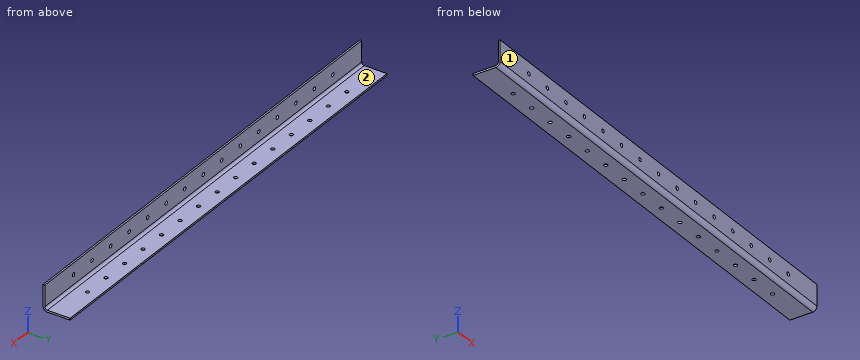
from build123d import *

# Parameters (mm, degrees)
SKETCH1_W                    = 2600
SKETCH1_H                    = 150
BASE_FLANGE1_DEPTH           = 10
EDGE_FLANGE1_STRIP_W         = 68
EDGE_FLANGE1_STRIP_H         = 10
EDGE_FLANGE1_STRIP_CUT_DEPTH = 2600
EDGE_FLANGE1_DEPTH           = 2600
SKETCH12_R                   = 10
CUT_EXTRUDE1_DEPTH           = 10
SKETCH13_R                   = 10
CUT_EXTRUDE2_DEPTH           = 10
LPATTERN1_COUNT              = 15
LPATTERN1_PITCH              = 152


# Sheet-metal steps are written as plain solids
with BuildPart() as part:
    # Sketch1 → Base-Flange1 (new body)
    with BuildSketch(Plane.XY):
        Rectangle(SKETCH1_W, SKETCH1_H)
    extrude(amount=-BASE_FLANGE1_DEPTH)

    # Edge-Flange1 strip (across the edge) → Edge-Flange1 strip cut (cut)
    with BuildSketch(Plane(origin=(-1300, -75, 0), x_dir=(0, 1, 0), z_dir=(1, 0, 0))):
        with Locations((-10, -5)):
            Rectangle(EDGE_FLANGE1_STRIP_W, EDGE_FLANGE1_STRIP_H)
    extrude(amount=EDGE_FLANGE1_STRIP_CUT_DEPTH, mode=Mode.SUBTRACT)

    # Edge-Flange1 section (across the edge) → Edge-Flange1 (add)
    with BuildSketch(Plane(origin=(-1300, -75, 0), x_dir=(0, 1, 0), z_dir=(1, 0, 0))):
        with BuildLine():
            Line((0, 14), (0, 130))
            Line((0, 130), (10, 130))
            Line((10, 130), (10, 14))
            ThreePointArc((10, 14), (14.100505063, 4.100505063), (24, 0))
            Line((24, 0), (24, -10))
            ThreePointArc((24, -10), (7.029437252, -2.970562748), (0, 14))
        make_face()
    extrude(amount=EDGE_FLANGE1_DEPTH)

    # Sketch12 → Cut-Extrude1 (cut)
    with BuildSketch(Plane(origin=(0, -75, 0), x_dir=(-1, 0, 0), z_dir=(0, -1, 0))):
        with Locations(Location((1064, -67, 0), (0, 0, 90))):
            Circle(SKETCH12_R)
    cut_extrude1 = extrude(amount=-CUT_EXTRUDE1_DEPTH, mode=Mode.SUBTRACT)

    # Sketch13 → Cut-Extrude2 (cut)
    with BuildSketch(Plane(origin=(0, 0, -10), x_dir=(-1, 0, 0), z_dir=(0, 0, -1))):
        with Locations((1064, 12)):
            Circle(SKETCH13_R)
    cut_extrude2 = extrude(amount=-CUT_EXTRUDE2_DEPTH, mode=Mode.SUBTRACT)

    # LPattern1: Cut-Extrude1, Cut-Extrude2 ×15
    with Locations(*[(i * LPATTERN1_PITCH, 0, 0) for i in range(1, LPATTERN1_COUNT)]):
        add(cut_extrude1, mode=Mode.SUBTRACT)
        add(cut_extrude2, mode=Mode.SUBTRACT)


solid = part.part
For this review, take the finished solid that the model builds, in its own axes (mm). Face numbers are marked on the shaded views. A direction names the side the tool comes from. Give positions to 0.01 mm unless a question says otherwise; leave off trailing zeros. Order: outer loops, then holes, each group sorted by start corner. A loop starts at its lowest first (then second) coordinate and runs counter-clockwise, first axis right, second up. Notation, with made-up numbers: M 21.5,43 L 28.5,43 A21 cw 28.5,67 Z; hole C 37,65.5 d6. An arc over 180 degrees is marked long. Answer in a Markdown table with one row per item. Add a question column.
(1) Wall thickness on probe 1 along Z at (x, y) = (-960, -25); probe 2 along Y at (x, z) = (868, 21.5); probe 3 along Y at (x, z) = (-912, -3): over which ranges is each line inside the solid? List them lowest first. Write a range as [from, to].
(2) Consider section A-A on x = 877. State the section outline as (y, z) points.
(3) Consider section B-B on y = -27. State the section outline as (x, z) points.
(4) For pin 1 (1.5 mm diameter, centred on x = 6, y = -52, fed in from -Z); pin 2 (18 mm diameter, centred on x = 760, y = 12, fed in from -Z); pin 3 (12 mm diameter, centred on x = 681.5, y = 31.5, fed in from +Z); pin 4 (23 mm diameter, centred on x = 608, z = 67, fed in from +Y), all flat-tipped, find the tip position at first contact; note any pin that passes through.
(5) For the marked faces 1 and 2, list the 3-axis set-ups (+Z, -Z, +X, -X, +Y, -Y) from which the entire face can be reached by the end or side of a thin tool; tool diameter is ignored.
Evaluation:
| question | item | result |
|---|---|---|
| 1 | probe 1 | z = [-10, 0] |
| 1 | probe 2 | y = [-75, -65] |
| 1 | probe 3 | y = [-67.94, 2], [22, 75] |
| 2 | outline | M -75,14 A24 ccw -51,-10 L 75,-10 L 75,0 L -51,0 A14 cw -65,14 L -65,130 L -75,130 Z |
| 3 | outline | M -1300,-10 L 1300,-10 L 1300,0 L -1300,0 Z |
| 4 | pin 1 | stops at z = -10 |
| 4 | pin 2 | passes through |
| 4 | pin 3 | stops at z = 0 |
| 4 | pin 4 | stops at y = -65 |
| 5 | face 1 | +Z, -Z, +X, -X, -Y |
| 5 | face 2 | +Z, +X, -X, +Y |
